Here's how the part is built. I have some questions about the finished solid (model axes, mm). A direction names the side the tool comes from. Round coordinates to 2 decimals unless told otherwise and drop trailing zeros. Order: outer loops, then holes, each group sorted by start corner. A loop starts at its lowest first (then second) coordinate and runs counter-clockwise, first axis right, second up.
```python
from build123d import *

# Parameters (mm, degrees)
CUT_EXTRUDE1_DEPTH = 24
SKETCH4_R          = 1.171537451
CUT_EXTRUDE2_DEPTH = 5.3


with BuildPart() as part:
    # Sketch2 → Revolve1 (revolve)
    with BuildSketch(Plane(origin=(0, 0, 0), x_dir=(0, 0, -1), z_dir=(1, 0, 0))):
        Polygon((0, 0), (0, 28), (-3, 28), (-3, 24), (-1.75, 24), (-1.75, 0), align=None)
    revolve(axis=Axis((0, 0, 0), (0, 1, 0)))

    # Sketch3 → Cut-Extrude1 (cut)
    with BuildSketch(Plane.XZ):
        with BuildLine():
            Line((-1.171537451, 1.3), (1.171537451, 1.3))
            ThreePointArc((1.171537451, 1.3), (0, 1.75), (-1.171537451, 1.3))
        make_face()
    extrude(amount=-CUT_EXTRUDE1_DEPTH, mode=Mode.SUBTRACT)

    # Sketch4 → Cut-Extrude2 (cut, through all)
    with BuildSketch(Plane.XY.offset(1.3)):
        with Locations((0, 2.5)):
            Circle(SKETCH4_R)
    extrude(amount=-CUT_EXTRUDE2_DEPTH, mode=Mode.SUBTRACT)


solid = part.part
```
1) For faces 1 (the flat face through (-2, 24, 0)), 2 (the flat face through (0, 1, 1.3)), 3 (the flat face through (0, 28, 0)), which set-ups out of +Z, -Z, +X, -X, +Y, -Y let a thin tool reach every point of the face, with its end or its side?
2) If we section it at D-D (z = -2.2): Write out the boundary of the cut face in (x, y).
3) If we section it at C-C (y = 22.75): Write out the boundary of the cut face in (x, z).
4) If we section it at A-A (x = 0): Write out the boundary of the cut face in (y, z).
5) I'm going to push flat-ended pins straight in: pin 1 (2 mm diameter, centred on y = 4, z = -1.5, fed in from +X); pin 2 (0.7 mm diameter, centred on x = 0.5, y = 1, fed in from +Z). Where does each tip first touch, or does it pass through?
6) If we section it at B-B (z = 0.8): Write out the boundary of the cut face in (x, y).
7) I need wall thicknesses on line 1 (Y direction, x = -0.1, z = 0.5); line 2 (X direction, y = 2.5, z = -0.05); line 3 (Y direction, x = -0.8, z = 1.55). Which ranges of each line are inside material? Lowest first, please.
8) We'd pull the mould along X, two halves only. Please class faces 4 (the flat face through (0, 13, 1.3)), 5 (the cylindrical face through (0.06, 11.83, -1.75)), 6 (the cylindrical face through (1.1, 2.9, -0.2)): +X half, -X half, draft (parallel to the pull), parting line (faces both ways), or undercut.
Solutions:
1. face 1: -Y
1. face 2: +Z, +X, -X, -Y
1. face 3: +Z, -Z, +X, -X, +Y
2. outline: (-2.04, 24) - (2.04, 24) - (2.04, 28) - (-2.04, 28) - close
3. outline: (-1.17, 1.3) arc R1.75 ccw (long way) to (1.17, 1.3) - close
4. outline: (0, -1.75) - (1.33, -1.75) - (1.33, 1.3) - (0, 1.3) - close; (3.67, -1.75) - (24, -1.75) - (24, -3) - (28, -3) - (28, 3) - (24, 3) - (24, 1.3) - (3.67, 1.3) - close
5. pin 1: stops at x = 1.68
5. pin 2: stops at z = 1.3
6. outline: (-2.89, 24) - (-1.56, 24) - (-1.56, 0) - (1.56, 0) - (1.56, 24) - (2.89, 24) - (2.89, 28) - (-2.89, 28) - close; hole circle Ø2.34 at (0, 2.5)
7. line 1: y = 0 to 1.33, 3.67 to 28
7. line 2: x = -1.75 to -1.17, 1.17 to 1.75
7. line 3: y = 24 to 28
8. face 4: draft
8. face 5: parting line
8. face 6: undercut
